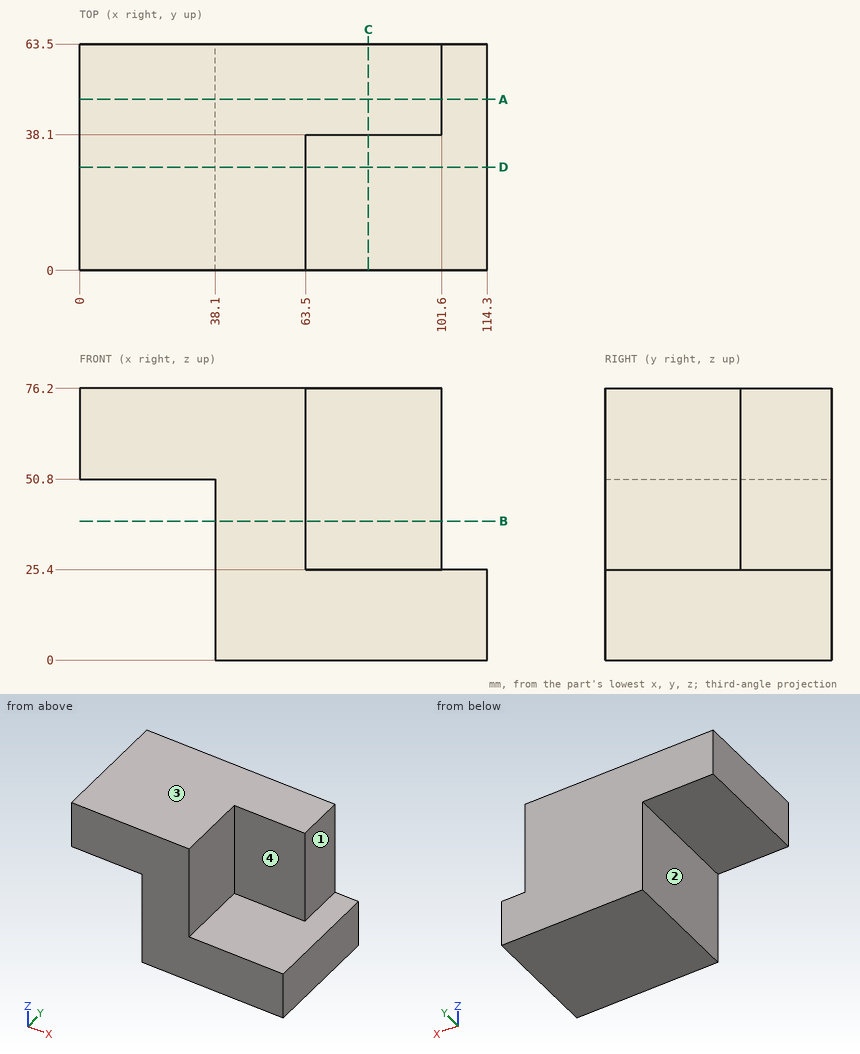
Source: three-view drawing plus pictorial views. Frame: mm from the lowest corner of the part. A direction names the side the tool comes from. Coordinates: 2 decimals unless noted, no trailing zeros. Write each loop counter-clockwise with the first axis right and the second up, starting at its lowest first coordinate (ties: lowest second). Pieces come first, ordered by that corner, then holes. Notation, with made-up numbers: (60.25, 52) - (110.25, 52) arc R31 ccw to (110.25, 80) - close; hole circle Ø2 at (65, 35.5). An arc over 180 degrees is marked (long way). Return JSON: item names as keys, results as strings.
Item 1: Line query: L1, parallel to Z at x = 86, y = 24; L2, parallel to Y at x = 91, z = 36; L3, parallel to Z at x = 20, y = 17. Output: solid intervals per line, ascending.
Completed:
{"L1": "z = 0 to 25.4", "L2": "y = 38.1 to 63.5", "L3": "z = 50.8 to 76.2"}
Item 2: Section query C-C (x = 81). Output: boundary loops of the cut face in (y, z).
Completed:
{"outline": "(0, 0) - (63.5, 0) - (63.5, 76.2) - (38.1, 76.2) - (38.1, 25.4) - (0, 25.4) - close"}
Item 3: Section query D-D (y = 29). Output: boundary loops of the cut face in (x, z).
Completed:
{"outline": "(0, 50.8) - (38.1, 50.8) - (38.1, 0) - (114.3, 0) - (114.3, 25.4) - (63.5, 25.4) - (63.5, 76.2) - (0, 76.2) - close"}
Item 4: Reachability of the marked faces 1, 2, 3 and 4 from +Z, -Z, +X, -X, +Y, -Y: full face, straight path, thin tool, end or side. Return the list, or none.
Completed:
{"face 1": "+Z, +X, +Y, -Y", "face 2": "-Z, -X, +Y, -Y", "face 3": "+Z, +X, -X, +Y, -Y", "face 4": "+Z, +X, -Y"}
Item 5: Pin query (flat end, axial travel): pin 1 Ø6 at (x, y) = (25.5, 55) entering from -Z; pin 2 Ø5 at (y, z) = (27, 64) entering from +X. Return the tip coordinate at first contact, or that it passes through.
Completed:
{"pin 1": "stops at z = 50.8", "pin 2": "stops at x = 63.5"}
Item 6: Section query A-A (y = 48). Output: boundary loops of the cut face in (x, z).
Completed:
{"outline": "(0, 50.8) - (38.1, 50.8) - (38.1, 0) - (114.3, 0) - (114.3, 25.4) - (101.6, 25.4) - (101.6, 76.2) - (0, 76.2) - close"}
Item 7: Section query B-B (z = 39). Output: boundary loops of the cut face in (x, y).
Completed:
{"outline": "(38.1, 0) - (63.5, 0) - (63.5, 38.1) - (101.6, 38.1) - (101.6, 63.5) - (38.1, 63.5) - close"}
